```python
from build123d import *

# Parameters (mm, degrees)
F0_R      = 9.9
F1_DEPTH  = 32
F0_W      = 37
F0_H      = 47
F2_DEPTH  = 25.8
F3_DEPTH  = 20
F5_SIZE2  = 20
F5_SIZE   = 2
F6_DEPTH  = 25.801
F8_DEPTH  = 57.001
F11_DEPTH = 57.001
F12_DEPTH = 25.801
F13_W     = 1.2
F13_H     = 9.9
F13_H_2   = 1.2
F13_W_2   = 9.9
F14_DEPTH = 25
F15_R     = 3


with BuildPart() as f1:
    # F0 (on Top) → F1 (new body)
    with BuildSketch(Plane.XY):
        Circle(F0_R)
    extrude(amount=F1_DEPTH)

    # F0 (on Top) → F2 (join)
    with BuildSketch(Plane.XY):
        Rectangle(F0_W, F0_H)
        Circle(F0_R, mode=Mode.SUBTRACT)
        Circle(F0_R)
    extrude(amount=-F2_DEPTH)

    # F3 (add): a face of the model
    f3_faces = [f1.faces().sort_by_distance(p)[0] for p in [
        (18.5, 0, -12.9),
    ]]
    extrude(f3_faces, amount=F3_DEPTH)

    # F5
    f5_edges = [f1.edges().sort_by_distance(p)[0] for p in [
        (-9.9, 0, 32),
    ]]
    f5_side = f1.faces().sort_by_distance((0, 0, 32))[0]
    chamfer(f5_edges, length=F5_SIZE, length2=F5_SIZE2, reference=f5_side)

    # F4 (on face) → F6 (cut, through all)
    with BuildSketch(Plane.XY):
        with BuildLine():
            Line((38.5, -15.1986841536), (38.5, 15.1986841536))
            ThreePointArc((38.5, 15.1986841536), (27.5, 0), (38.5, -15.1986841536))
        make_face()
    extrude(amount=-F6_DEPTH, mode=Mode.SUBTRACT)

    # F7 (on face) → F8 (cut, through all)
    with BuildSketch(Plane(origin=(-18.5, 0, 0), x_dir=(0, -1, 0), z_dir=(-1, 0, 0))):
        Polygon((-23.5, -16.9), (-19.027864045, -12.9), (-23.5, -8.9), align=None)
        Polygon((19.027864045, -12.9), (23.5, -16.9), (23.5, -8.9), align=None)
    extrude(amount=-F8_DEPTH, mode=Mode.SUBTRACT)

    # F10 (on face) → F11 (cut, through all)
    with BuildSketch(Plane(origin=(-18.5, 0, 0), x_dir=(0, -1, 0), z_dir=(-1, 0, 0))):
        Polygon((4, -25.8), (0, -21.327864045), (-4, -25.8), align=None)
    extrude(amount=-F11_DEPTH, mode=Mode.SUBTRACT)

    # F9 (on face) → F12 (cut, through all)
    with BuildSketch(Plane.XY):
        Polygon((-18.5, -4), (-14.027864045, 0), (-18.5, 4), align=None)
    extrude(amount=-F12_DEPTH, mode=Mode.SUBTRACT)

    # F13 (on face) → F14 (cut)
    with BuildSketch(Plane.XY.offset(32)):
        with Locations((0, -5.55)):
            Rectangle(F13_W, F13_H)
        Rectangle(F13_W, F13_H_2)
        with Locations((5.55, 0)):
            Rectangle(F13_W_2, F13_H_2)
        with Locations((-5.55, 0)):
            Rectangle(F13_W_2, F13_H_2)
        with Locations((0, 5.55)):
            Rectangle(F13_W, F13_H)
    extrude(amount=-F14_DEPTH, mode=Mode.SUBTRACT)

    # F15
    f15_edges = [f1.edges().sort_by_distance(p)[0] for p in [
        (-18.5, 23.5, -4.45),
        (-18.5, 23.5, -21.35),
        (-18.5, -23.5, -4.45),
        (-18.5, -23.5, -21.35),
        (38.5, -23.5, -4.45),
        (38.5, -23.5, -21.35),
        (38.5, 15.198684, -12.9),
        (38.5, -15.198684, -12.9),
        (38.5, 23.5, -4.45),
        (38.5, 23.5, -21.35),
        (10, -23.5, 0),
        (10, 23.5, 0),
        (10, 23.5, -16.9),
        (10, -23.5, -8.9),
        (10, -23.5, -16.9),
        (10, 23.5, -8.9),
        (-18.5, 4, -12.9),
        (-18.5, -4, -12.9),
        (-5.586144, 5.586144, 32),
        (-5.586144, -5.586144, 32),
        (5.586144, -5.586144, 32),
        (5.586144, 5.586144, 32),
    ]]
    fillet(f15_edges, radius=F15_R)


solid = f1.part
```
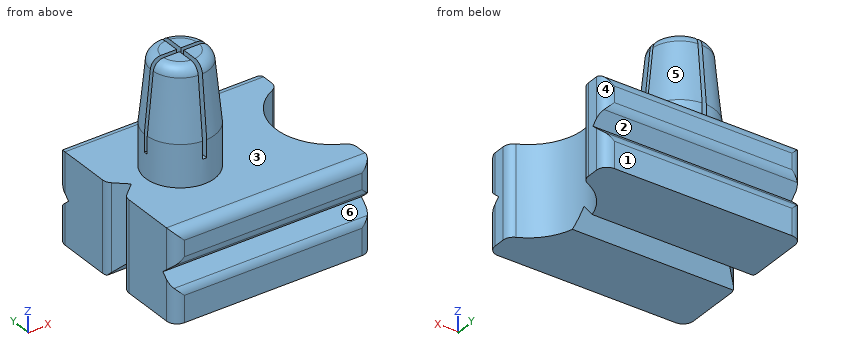
Can you work these out from the model? Positions are in its coordinate system, mm. Face numbers are marked on the shaded views. A direction names the side the tool comes from. Give positions to 0.01 mm unless a question says otherwise; leave off trailing zeros. Order: outer loops, then holes, each group sorted by start corner. A loop starts at its lowest first (then second) coordinate and runs counter-clockwise, first axis right, second up. Notation, with made-up numbers: (28, 56.5) - (84, 56.5) arc R7 ccw to (84, 67.5) - close; hole circle Ø3 at (14, -35). An arc over 180 degrees is marked (long way). Use a Markdown table: item, result. Add a question column.
Q1. If we mould it in two halves opening along Z, with no side actions, what happens to the marked faces 4, 5 and 6? For each: released by +Z, released by -Z, zero draft, split by the parting line, or undercut.
Q2. I'm going to push flat-ended pins straight in: pin 1 (10 mm diameter, centred on y = 6.5, z = 21, fed in from +X); pin 2 (10 mm diameter, centred on y = -11, z = -15, fed in from +X); pin 3 (6 mm diameter, centred on y = 3.5, z = -5.5, fed in from +X). Where does each tip first touch, or does it pass through?
Q3. If we section it at B-B on z = 16.5: Write out the boundary of the cut face in (x, y), plus the area to 3 significant figures.
Q4. If we section it at A-A on x = 15: Write out the boundary of the cut face in (y, z), plus the area to 3 significant figures.
Q5. Please list where these lines run through material, in increasing order: line 1 along Z through (x, y) = (21, 17); line 2 along Y through (x, z) = (1, 20.5); line 3 along Z through (x, y) = (0, 9.5).
Q6. On a 3-axis mill with a long thin cutter (end or side, diameter ignored), from which of +Z, -Z, +X, -X, +Y, -Y can I reach the whole of each face in a straight line? I mean the marked faces 1, 2 and 3. Say none if no direction works.
Q7. If we section it at C-C on x = 31.5: Write out the boundary of the cut face in (y, z), plus the area to 3 significant figures.
Q8. If we section it at D-D on z = -20.5: Write out the boundary of the cut face in (x, y).
Answers follow:
| question | item | result |
|---|---|---|
| 1 | face 4 | zero draft |
| 1 | face 5 | released by +Z |
| 1 | face 6 | undercut |
| 2 | pin 1 | stops at x = 9 |
| 2 | pin 2 | stops at x = 38.23 |
| 2 | pin 3 | stops at x = 28.88 |
| 3 | outline | (-9.43, -0.6) arc R9.45 ccw to (-0.6, -9.43) - (-0.6, -0.6) - close; (-9.43, 0.6) - (-0.6, 0.6) - (-0.6, 9.43) arc R9.45 ccw to start; (0.6, -9.43) arc R9.45 ccw to (9.43, -0.6) - (0.6, -0.6) - close; (0.6, 0.6) - (9.43, 0.6) arc R9.45 ccw to (0.6, 9.43) - close |
| 3 | area | 237 mm^2 |
| 4 | outline | (-23.5, -25.8) - (-4, -25.8) - (0, -21.33) - (4, -25.8) - (23.5, -25.8) - (23.5, -18.24) arc R3 ccw to (22.5, -16.01) - (19.03, -12.9) - (22.5, -9.79) arc R3 ccw to (23.5, -7.56) - (23.5, -3) arc R3 ccw to (20.5, 0) - (-20.5, 0) arc R3 ccw to (-23.5, -3) - (-23.5, -7.56) arc R3 ccw to (-22.5, -9.79) - (-19.03, -12.9) - (-22.5, -16.01) arc R3 ccw to (-23.5, -18.24) - close |
| 4 | area | 1,150 mm^2 |
| 5 | line 1 | z = -25.8 to 0 |
| 5 | line 2 | y = -8.99 to -0.6, 0.6 to 8.99 |
| 5 | line 3 | z = -25.8 to 7 |
| 6 | face 1 | +Z, -Z, +X, -X, +Y |
| 6 | face 2 | +X, -X, +Y |
| 6 | face 3 | +Z |
| 7 | outline | (-23.5, -25.8) - (-10.58, -25.8) - (-10.58, 0) - (-20.5, 0) arc R3 ccw to (-23.5, -3) - (-23.5, -7.56) arc R3 ccw to (-22.5, -9.79) - (-19.03, -12.9) - (-22.5, -16.01) arc R3 ccw to (-23.5, -18.24) - close; (10.58, -25.8) - (23.5, -25.8) - (23.5, -18.24) arc R3 ccw to (22.5, -16.01) - (19.03, -12.9) - (22.5, -9.79) arc R3 ccw to (23.5, -7.56) - (23.5, -3) arc R3 ccw to (20.5, 0) - (10.58, 0) - close |
| 7 | area | 626 mm^2 |
| 8 | outline | (-18.5, -20.5) arc R3 ccw to (-15.5, -23.5) - (35.5, -23.5) arc R3 ccw to (38.5, -20.5) - (38.5, -17.23) arc R3 ccw to (36.76, -14.51) arc R16 cw to (36.76, 14.51) arc R3 ccw to (38.5, 17.23) - (38.5, 20.5) arc R3 ccw to (35.5, 23.5) - (-15.5, 23.5) arc R3 ccw to (-18.5, 20.5) - (-18.5, 5.34) arc R3 ccw to (-17.5, 3.11) - (-14.03, 0) - (-17.5, -3.11) arc R3 ccw to (-18.5, -5.34) - close |
